from build123d import *

# Parameters (mm, degrees)
SKETCH1_W           = 65
SKETCH1_H           = 51
BOSS_EXTRUDE1_DEPTH = 3
SKETCH3_W           = 6.75
SKETCH3_H           = 6.15
CUT_EXTRUDE1_DEPTH  = 4
SKETCH4_W           = 2.5
SKETCH4_H           = 9
CUT_EXTRUDE2_DEPTH  = 4


with BuildPart() as part:
    # Sketch1 → Boss-Extrude1 (new body)
    with BuildSketch(Plane.XY):
        with Locations((-744.213414634, 1009.240243902)):
            Rectangle(SKETCH1_W, SKETCH1_H)
    extrude(amount=BOSS_EXTRUDE1_DEPTH)

    # Sketch3 → Cut-Extrude1 (cut, through all)
    with BuildSketch(Plane.XY.offset(3)):
        with Locations((-773.338414634, 986.815243902)):
            Rectangle(SKETCH3_W, SKETCH3_H)
        with Locations((-715.088414634, 986.815243902)):
            Rectangle(SKETCH3_W, SKETCH3_H)
    extrude(amount=-CUT_EXTRUDE1_DEPTH, mode=Mode.SUBTRACT)

    # Sketch4 → Cut-Extrude2 (cut, through all)
    with BuildSketch(Plane.XY.offset(3)):
        Polygon((-761.516384975, 1007.624918562), (-761.516384975, 1016.624918562), (-764.016384975, 1016.624918562), (-764.016384975, 998.624918562), (-759.016384975, 998.624918562), (-759.016384975, 1007.624918562), align=None)
        with Locations((-760.266384975, 1012.124918562)):
            Rectangle(SKETCH4_W, SKETCH4_H)
        Polygon((-724.410444293, 1016.624918562), (-726.910444293, 1016.624918562), (-726.910444293, 1007.624918562), (-729.410444293, 1007.624918562), (-729.410444293, 998.624918562), (-724.410444293, 998.624918562), align=None)
        with Locations((-728.160444293, 1012.124918562)):
            Rectangle(SKETCH4_W, SKETCH4_H)
    extrude(amount=-CUT_EXTRUDE2_DEPTH, mode=Mode.SUBTRACT)


solid = part.part
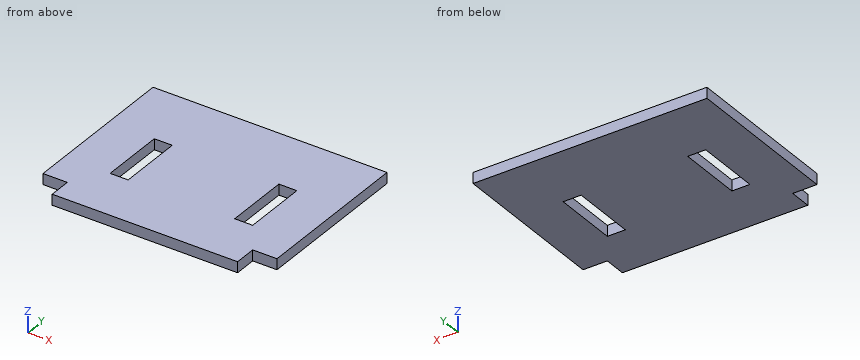
Input: part model. Units: mm. Frame: model coordinates. Give positions to 0.01 mm unless a question says otherwise; leave off trailing zeros. Loops run counter-clockwise (first coordinate to the right, second up) from the corner with the lowest first, then second, coordinate; pieces in that order, holes last. Notation, with made-up numbers: (78.5, -11) - (117.5, -11) arc R15 ccw to (117.5, 12) - close; hole circle Ø4 at (-30.75, 36.25). An arc over 180 degrees is marked (long way). Use CSV: the item, a comma, the result in double quotes. Start each with the question number.
Item 1: Section B-B on x = -726.5. Return loops of the section in (y, z), then the cut area to 3 significant figures.
Item 2: Line query: line 1 (X direction, y = 1013, z = 0.6); line 2 (Y direction, x = -761.5, z = 0.7); line 3 (Y direction, x = -713.5, z = 0.8). Output: solid intervals per line, ascending.
Item 3: Section C-C on z = 0.45. Return loops of the section in (x, y).
Item 4: Section A-A on y = 1012. Return loops of the section in (x, z).
Ans:
1,outline,"(983.74, 0) - (998.62, 0) - (998.62, 3) - (983.74, 3) - close; (1016.62, 0) - (1034.74, 0) - (1034.74, 3) - (1016.62, 3) - close"
1,area,"99.0 mm2"
2,line 1,"x = -776.71 to -764.02, -759.02 to -729.41, -724.41 to -711.71"
2,line 2,"y = 983.74 to 998.62, 1016.62 to 1034.74"
2,line 3,"y = 989.89 to 1034.74"
3,outline,"(-776.71, 989.89) - (-769.96, 989.89) - (-769.96, 983.74) - (-718.46, 983.74) - (-718.46, 989.89) - (-711.71, 989.89) - (-711.71, 1034.74) - (-776.71, 1034.74) - close; hole (-764.02, 998.62) - (-759.02, 998.62) - (-759.02, 1016.62) - (-764.02, 1016.62) - close; hole (-729.41, 998.62) - (-724.41, 998.62) - (-724.41, 1016.62) - (-729.41, 1016.62) - close"
4,outline,"(-776.71, 0) - (-764.02, 0) - (-764.02, 3) - (-776.71, 3) - close; (-759.02, 0) - (-729.41, 0) - (-729.41, 3) - (-759.02, 3) - close; (-724.41, 0) - (-711.71, 0) - (-711.71, 3) - (-724.41, 3) - close"
